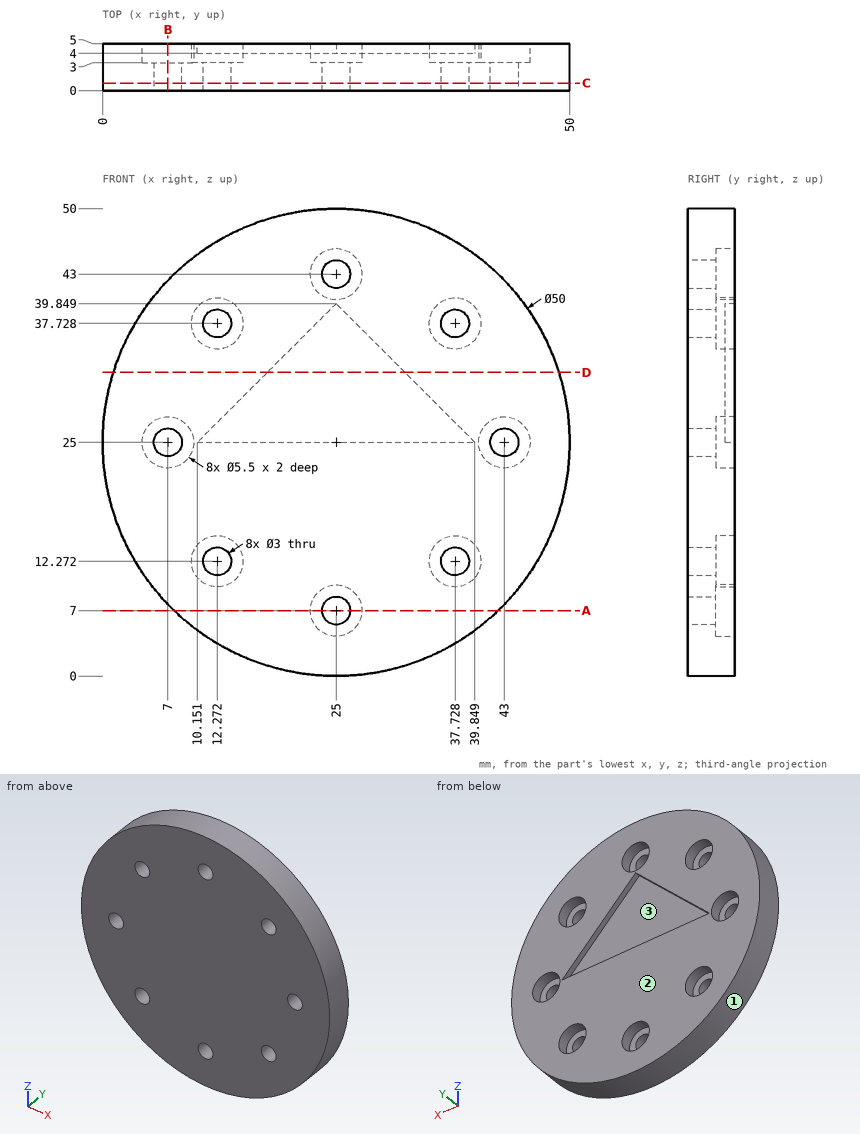
Answer from the drawing. Dimensions are ordinates in mm from the lowest x, y and z of the part. Coordinates: 2 decimals unless noted, no trailing zeros. Order: outer loops, then holes, each group sorted by start corner. A loop starts at its lowest first (then second) coordinate and runs counter-clockwise, first axis right, second up. Notation, with made-up numbers: (47.25, 7) - (75.25, 7) arc R12 ccw to (75.25, 12) - close; hole circle Ø10 at (-10.75, -1). An arc over 180 degrees is marked (long way). Use one line per item in the form item = value.
(1) Given pin 1 Ø4 at (x, z) = (25, 7) entering from -Y; pin 2 Ø3 at (y, z) = (2, 34.5) entering from +X (1 decimal); pin 3 Ø3 at (x, z) = (24.5, 42) entering from +Y; pin 4 Ø2.5 at (x, z) = (12.27, 37.73) entering from -Y, each flat-ended and moving along its own axis, determine where each tip first touches the part or whether it passes through.
Computed values:
pin_1 = 0
pin_2 = 48.7
pin_3 = 3
pin_4 = through
(2) Section C-C, the plane y = 0.8 is taken. Give the number of separate pieces and of enclosed holes in the cut face, then the cut area to 3 significant figures.
Computed values:
separate_pieces = 1
enclosed_holes = 8
area = 1,910 mm²
(3) Straight lines are drawn through the part: L1, parallel to Z at x = 24.5, y = 1 (1 decimal); L2, parallel to X at y = 1.7, z = 43; L3, parallel to Y at x = 17, z = 26. For each, find the intervals that lie inside material, in ascending order.
Computed values:
L1 = 0 to 5.6, 8.4 to 41.6, 44.4 to 50
L2 = 7.65 to 23.5, 26.5 to 42.35
L3 = 0 to 4
(4) Section A-A, the plane z = 7 is taken. Give the vertices of the cut face in (x, y), then the cut area to 4 significant figures.
Computed values:
outline = (7.65, 0) - (23.5, 0) - (23.5, 3) - (22.25, 3) - (22.25, 5) - (7.65, 5) - close; (26.5, 0) - (42.35, 0) - (42.35, 5) - (27.75, 5) - (27.75, 3) - (26.5, 3) - close
area = 153.5 mm²
(5) For a pull along X with two mould halves and no side action, classify the marked faces 1, 2 and 3 as pulls with the +X half, pulls with the -X half, needs draft (parallel to the pull), parting line crosses it, or undercut.
Computed values:
face_1 = parting line crosses it
face_2 = needs draft
face_3 = undercut
(6) Section D-D, the plane z = 32.5 is taken. Give the vertices of the cut face in (x, y), then the cut area to 3 significant figures.
Computed values:
outline = (1.15, 0) - (48.85, 0) - (48.85, 5) - (32.35, 5) - (32.35, 4) - (17.65, 4) - (17.65, 5) - (1.15, 5) - close
area = 224 mm²
(7) Section B-B, the plane x = 7 is taken. Give the vertices of the cut face in (y, z), then the cut area to 4 significant figures.
Computed values:
outline = (0, 7.65) - (5, 7.65) - (5, 22.25) - (3, 22.25) - (3, 23.5) - (0, 23.5) - close; (0, 26.5) - (3, 26.5) - (3, 27.75) - (5, 27.75) - (5, 42.35) - (0, 42.35) - close
area = 153.5 mm²
